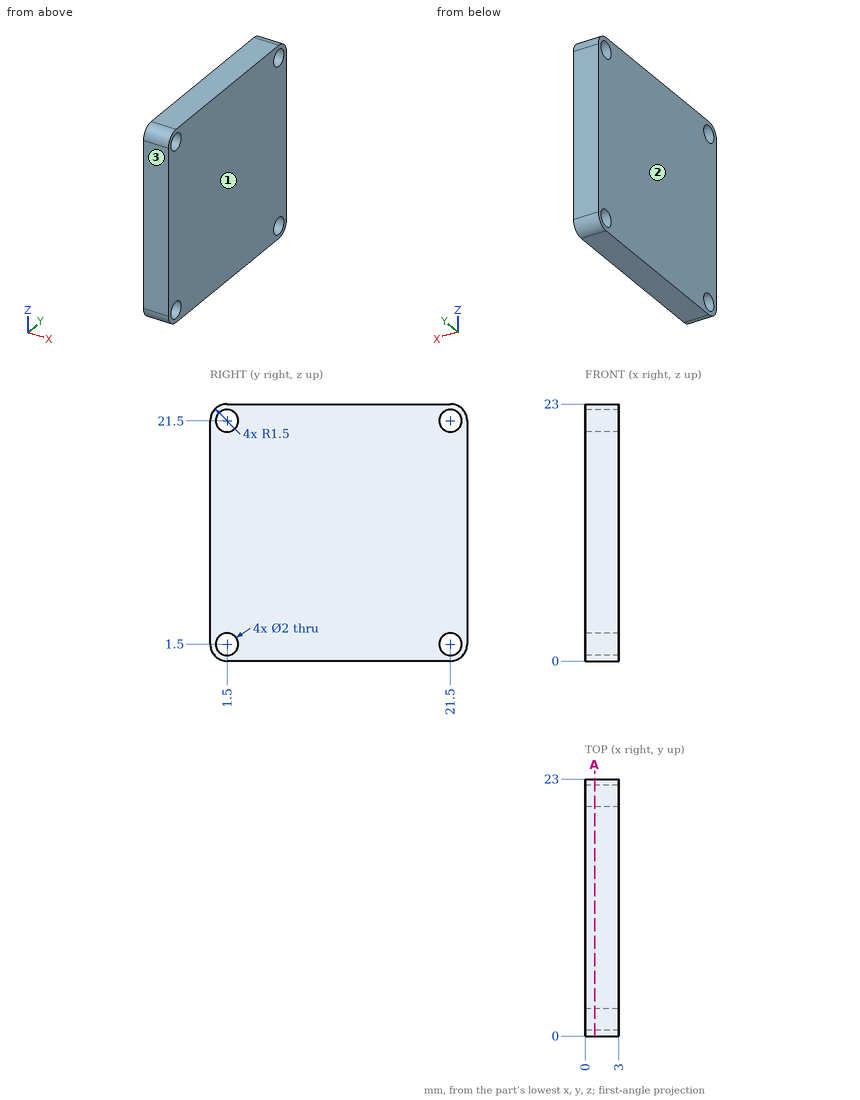
Study the drawing (mm; zero at the part's minimum x, y, z) and answer. Give positions to 0.01 mm unless a question says otherwise; leave off trailing zeros. Loops run counter-clockwise (first coordinate to the right, second up) from the corner with the lowest first, then second, coordinate; pieces in that order, holes last. Notation, with made-up numbers: (45, 1) -> (71, 1) arc R18 ccw to (71, 30) -> close; hole circle Ø4 at (-11, 39.25). An arc over 180 degrees is marked (long way). Use a Markdown table: item, result. Add a question column.
1) For a pull along X with two mould halves and no side action, classify the marked faces 1, 2 and 3 as +X half, -X half, draft (parallel to the pull), parting line (faces both ways), or undercut.
2) The part is cut by section A-A, the plane x = 0.85. Determine the outline of the cut face in (y, z).
3) Consider line 1 along Z through (x, y) = (2.25, 1.5). Determine where the line is inside the solid, lowest interval first.
Reported:
| question | item | result |
|---|---|---|
| 1 | face 1 | +X half |
| 1 | face 2 | -X half |
| 1 | face 3 | draft |
| 2 | outline | (0, 1.5) arc R1.5 ccw to (1.5, 0) -> (21.5, 0) arc R1.5 ccw to (23, 1.5) -> (23, 21.5) arc R1.5 ccw to (21.5, 23) -> (1.5, 23) arc R1.5 ccw to (0, 21.5) -> close; hole circle Ø2 at (1.5, 1.5); hole circle Ø2 at (1.5, 21.5); hole circle Ø2 at (21.5, 1.5); hole circle Ø2 at (21.5, 21.5) |
| 3 | line 1 | z = 0 to 0.5, 2.5 to 20.5, 22.5 to 23 |
